For this review, take the finished solid that the model builds, in its own axes (mm). A direction names the side the tool comes from. Coordinates: 2 decimals unless noted, no trailing zeros. Loops run counter-clockwise (first coordinate to the right, second up) from the corner with the lowest first, then second, coordinate; pieces in that order, holes last. Notation, with made-up numbers: (35, -15) -> (78, -15) arc R23 ccw to (78, 3) -> close; hole circle Ø3 at (-26, 39.5). An arc over 180 degrees is marked (long way). Use a Markdown table: item, result.
from build123d import *

# Parameters (mm, degrees)
SKETCH1_W            = 54.61
SKETCH1_H            = 47.244
SKETCH1_W_2          = 41.91
SKETCH1_H_2          = 21.844
BOSS_EXTRUDE1_DEPTH  = 5.08
SKETCH2_R            = 0.93599
CUT_EXTRUDE1_DEPTH   = 73.388217522
SKETCH10_W           = 14.41958
SKETCH10_H           = 19.49958
SKETCH10_R           = 0.635
BOSS_EXTRUDE4_DEPTH  = 5.08
SKETCH11_R           = 0.635
SKETCH11_W           = 3.302
SKETCH11_H           = 76.2
BOSS_EXTRUDE5_DEPTH  = 5.08
SKETCH12_W           = 60.452
SKETCH12_H           = 6.35
SKETCH12_W_2         = 59.182
CUT_EXTRUDE2_DEPTH   = 95.448366629
SKETCH13_W           = 7.0195552
SKETCH13_H           = 78.993394517
BOSS_EXTRUDE6_DEPTH  = 4.826
FILLET1_R            = 2.54
CUT_EXTRUDE3_DEPTH   = 95.448366629
SKETCH15_W           = 9.078627065
SKETCH15_H           = 34.544
BOSS_EXTRUDE7_DEPTH  = 5.08
SKETCH16_W           = 10.16
SKETCH16_H           = 6.35
BOSS_EXTRUDE8_DEPTH  = 10.16
SKETCH19_W           = 41.91
SKETCH19_H           = 6.35
BOSS_EXTRUDE10_DEPTH = 44.45
SKETCH20_W           = 16.24457
SKETCH20_H           = 10.16
BOSS_EXTRUDE11_DEPTH = 6.35
SKETCH17_R           = 0.635
CUT_EXTRUDE4_DEPTH   = 88.397462588
SKETCH21_R           = 0.635
CUT_EXTRUDE5_DEPTH   = 89.359200918


with BuildPart() as part:
    # Sketch1 → Boss-Extrude1 (new body)
    with BuildSketch(Plane.XY):
        with Locations((27.305, 23.622)):
            Rectangle(SKETCH1_W, SKETCH1_H)
        with Locations((27.305, 23.622)):
            Rectangle(SKETCH1_W_2, SKETCH1_H_2, mode=Mode.SUBTRACT)
    extrude(amount=BOSS_EXTRUDE1_DEPTH)

    # Sketch2 → Cut-Extrude1 (cut, through all)
    with BuildSketch(Plane.XY.offset(5.08)):
        with Locations((2.80543, 28.62199)):
            Circle(SKETCH2_R)
        with Locations((2.80543, 18.62201)):
            Circle(SKETCH2_R)
        with Locations((51.80457, 28.62199)):
            Circle(SKETCH2_R)
        with Locations((51.80457, 18.62201)):
            Circle(SKETCH2_R)
    extrude(amount=-CUT_EXTRUDE1_DEPTH, mode=Mode.SUBTRACT)

    # Sketch10 → Boss-Extrude4 (add)
    with BuildSketch(Plane.XY.offset(5.08)):
        with Locations((61.81979, 23.622)):
            Rectangle(SKETCH10_W, SKETCH10_H)
        with Locations((64.35979, 21.49221)):
            Circle(SKETCH10_R, mode=Mode.SUBTRACT)
        with Locations((64.35979, 25.75179)):
            Circle(SKETCH10_R, mode=Mode.SUBTRACT)
    extrude(amount=-BOSS_EXTRUDE4_DEPTH)

    # Sketch11 → Boss-Extrude5 (add)
    with BuildSketch(Plane.XY.offset(5.08)):
        Polygon((0, 47.244), (-5.842, 47.244), (-5.842, 64.262), (-15.748, 64.262), (-15.748, -17.018), (-4.572, -17.018), (-4.572, 0), (0, 0), align=None)
        with Locations(Location((-4.572, 21.49221, 0), (0, 0, 180))):
            Circle(SKETCH11_R, mode=Mode.SUBTRACT)
        with Locations(Location((-4.572, 25.75179, 0), (0, 0, 180))):
            Circle(SKETCH11_R, mode=Mode.SUBTRACT)
        with Locations((-10.795, 23.622)):
            Rectangle(SKETCH11_W, SKETCH11_H, mode=Mode.SUBTRACT)
    extrude(amount=-BOSS_EXTRUDE5_DEPTH)

    # Sketch12 → Cut-Extrude2 (cut, through all)
    with BuildSketch(Plane.XY.offset(5.08)):
        with Locations((24.384, 44.069)):
            Rectangle(SKETCH12_W, SKETCH12_H)
        with Locations((25.019, 3.175)):
            Rectangle(SKETCH12_W_2, SKETCH12_H)
    extrude(amount=-CUT_EXTRUDE2_DEPTH, mode=Mode.SUBTRACT)

    # Sketch13 → Boss-Extrude6 (add)
    with BuildSketch(Plane(origin=(0, 0, 0), x_dir=(-1, 0, 0), z_dir=(0, 0, -1))):
        with Locations((10.665198327, 23.388014827)):
            Rectangle(SKETCH13_W, SKETCH13_H)
    extrude(amount=-BOSS_EXTRUDE6_DEPTH)

    # Fillet1
    fillet1_edges = [part.edges().sort_by_distance(p)[0] for p in [
        (69.02958, 13.87221, 2.54),
        (54.61, 13.87221, 2.54),
        (54.61, 6.35, 2.54),
        (-4.572, 6.35, 2.54),
        (-4.572, -17.018, 2.54),
        (-15.748, -17.018, 2.54),
        (-15.748, 64.262, 2.54),
        (-5.842, 64.262, 2.54),
        (-5.842, 40.894, 2.54),
        (54.61, 40.894, 2.54),
        (54.61, 33.37179, 2.54),
        (69.02958, 33.37179, 2.54),
    ]]
    fillet(fillet1_edges, radius=FILLET1_R)

    # Sketch14 → Cut-Extrude3 (cut, through all)
    with BuildSketch(Plane.XY.offset(5.08)):
        Polygon((2.80543, 40.894), (-0.815942935, 40.894), (-0.815942935, 6.35), (2.80543, 6.35), (2.80543, -19.941776761), (-23.515321153, -19.941776761), (-23.515321153, 65.826532556), (2.80543, 65.826532556), align=None)
        Polygon((51.80457, 40.896870143), (51.80457, 65.826532556), (74.486186006, 65.826532556), (74.486186006, -19.941776761), (51.80457, -19.941776761), (52.07, 6.35), (54.61, 8.89), (54.61, 38.354), align=None)
    extrude(amount=-CUT_EXTRUDE3_DEPTH, mode=Mode.SUBTRACT)

    # Sketch15 → Boss-Extrude7 (add)
    with BuildSketch(Plane.XY.offset(5.08)):
        with Locations((-5.355256468, 23.622)):
            Rectangle(SKETCH15_W, SKETCH15_H)
        Polygon((51.807736495, 40.894), (54.61, 38.354), (54.61, 8.89), (52.07, 6.35), (64.50457, 6.35), (64.50457, 40.894), align=None)
    extrude(amount=-BOSS_EXTRUDE7_DEPTH)

    # Sketch16 → Boss-Extrude8 (add)
    with BuildSketch(Plane.XY.offset(5.08)):
        with Locations((-4.81457, 35.179)):
            Rectangle(SKETCH16_W, SKETCH16_H)
        with Locations((59.42457, 35.179)):
            Rectangle(SKETCH16_W, SKETCH16_H)
    extrude(amount=BOSS_EXTRUDE8_DEPTH)

    # Sketch19 → Boss-Extrude10 (add)
    with BuildSketch(Plane.XY.offset(5.08)):
        with Locations((27.305, 9.525)):
            Rectangle(SKETCH19_W, SKETCH19_H)
    extrude(amount=BOSS_EXTRUDE10_DEPTH)

    # Sketch20 → Boss-Extrude11 (add)
    with BuildSketch(Plane(origin=(0, 6.35, 0), x_dir=(-1, 0, 0), z_dir=(0, -1, 0))):
        with Locations((1.772285, -10.16)):
            Rectangle(SKETCH20_W, SKETCH20_H)
        with Locations((-56.382285, -10.16)):
            Rectangle(SKETCH20_W, SKETCH20_H)
    extrude(amount=-BOSS_EXTRUDE11_DEPTH)

    # Sketch17 → Cut-Extrude4 (cut, through all)
    with BuildSketch(Plane(origin=(0, 38.354, 0), x_dir=(1, 0, 0), z_dir=(0, 1, 0))):
        with Locations(Location((-4.81457, -10.16, 0), (0, 0, 180))):
            Circle(SKETCH17_R)
        with Locations(Location((59.42457, -10.16, 0), (0, 0, 270))):
            Circle(SKETCH17_R)
    extrude(amount=-CUT_EXTRUDE4_DEPTH, mode=Mode.SUBTRACT)

    # Sketch21 → Cut-Extrude5 (cut, through all)
    with BuildSketch(Plane.XZ.offset(-6.35)):
        with Locations(Location((37.592, 23.241, 0), (0, 0, 270))):
            Circle(SKETCH21_R)
        with Locations(Location((37.592, 44.831, 0), (0, 0, 270))):
            Circle(SKETCH21_R)
        with Locations(Location((12.192, 44.831, 0), (0, 0, 270))):
            Circle(SKETCH21_R)
        with Locations(Location((12.192, 23.241, 0), (0, 0, 270))):
            Circle(SKETCH21_R)
    extrude(amount=-CUT_EXTRUDE5_DEPTH, mode=Mode.SUBTRACT)


solid = part.part
(1) Take a section at A-A on x = 30. Write out the cut boundary in (y, z).
Found:
| item | result |
|---|---|
| outline | (6.35, 0) -> (12.7, 0) -> (12.7, 49.53) -> (6.35, 49.53) -> close; (34.54, 0) -> (40.89, 0) -> (40.89, 5.08) -> (34.54, 5.08) -> close |
(2) For line 1 along X through (y, z) = (33, 4.5); line 2 along X through (y, z) = (34, 10); line 3 along X through (y, z) = (37.5, 12.5), list the stretches that pass through material, from the lowest coordinate up.
Found:
| item | result |
|---|---|
| line 1 | x = -9.89 to 6.35, 48.26 to 64.5 |
| line 2 | x = -9.89 to -5.43, -4.2 to 0.27, 54.34 to 58.81, 60.04 to 64.5 |
| line 3 | x = -9.89 to 0.27, 54.34 to 64.5 |
(3) Take a section at B-B on y = 23.5. Write out the cut boundary in (x, z).
Found:
| item | result |
|---|---|
| outline | (-9.89, 0) -> (6.35, 0) -> (6.35, 5.08) -> (-9.89, 5.08) -> close; (48.26, 0) -> (64.5, 0) -> (64.5, 5.08) -> (48.26, 5.08) -> close |
(4) Take a section at D-D on z = 31.5. Write out the cut boundary in (x, y), plus the area to 3 significant figures.
Found:
| item | result |
|---|---|
| outline | (6.35, 6.35) -> (48.26, 6.35) -> (48.26, 12.7) -> (6.35, 12.7) -> close |
| area | 266 mm^2 |
(5) For faces 1 (the face through (0.265, 35, 10)), 2 (the face through (6.35, 9, 32)), 3 (the face through (60.5, 38.354, 10.1)), list the 3-axis set-ups (+Z, -Z, +X, -X, +Y, -Y) from which the entire face can be reached by the end or side of a thin tool; tool diameter is ignored.
Found:
| item | result |
|---|---|
| face 1 | +Z, +Y |
| face 2 | +Z, -X, +Y, -Y |
| face 3 | +Z, +X, -X, +Y |
(6) Mouldability with a two-part tool opening along X and no side actions: class faces 4 (the face through (48.26, 9, 32)), 5 (the face through (51.062, 28.052, 2.576)), 6 (the face through (-2, 9, 15.24)) as pulls with the +X half, pulls with the -X half, needs draft (parallel to the pull), parting line crosses it, or undercut.
Found:
| item | result |
|---|---|
| face 4 | pulls with the +X half |
| face 5 | undercut |
| face 6 | needs draft |
(7) Take a section at C-C on x = -2.5. Write out the cut boundary in (y, z), plus the area to 3 significant figures.
Found:
| item | result |
|---|---|
| outline | (6.35, 0) -> (40.89, 0) -> (40.89, 5.08) -> (38.35, 5.08) -> (38.35, 15.24) -> (32, 15.24) -> (32, 5.08) -> (12.7, 5.08) -> (12.7, 15.24) -> (6.35, 15.24) -> close |
| area | 305 mm^2 |
(8) For pin 1 Ø25 at (x, z) = (15.5, 30) entering from +Y; pin 2 Ø3 at (x, y) = (51.8, 18.62) entering from +Z; pin 3 Ø1.9 at (x, y) = (-2.5, 36.5) entering from +Z, all flat-tipped, find the tip position at first contact; note any pin that passes through.
Found:
| item | result |
|---|---|
| pin 1 | stops at y = 12.7 |
| pin 2 | stops at z = 5.08 |
| pin 3 | stops at z = 15.24 |
